CAD build for the part. Positions are in the model's coordinates, mm. A direction names the side the tool comes from. Give positions to 0.01 mm unless a question says otherwise; leave off trailing zeros. Write each loop counter-clockwise with the first axis right and the second up, starting at its lowest first coordinate (ties: lowest second). Pieces come first, ordered by that corner, then holes. Notation, with made-up numbers: (-21, 6.25) - (23, 6.25) arc R24 ccw to (23, 29.25) - close; hole circle Ø3 at (-10, -16). An arc over 180 degrees is marked (long way). Put each result on its own line as item: value. Start each with the question number.
1. Mould opens along Y. For faces 1 (the cylindrical face through (79.47, -0.8, 24.65)), 2 (the flat face through (-100.519, -2, 25)), 3 (the flat face through (-34, 48.316, 25)), 4 (the flat face through (-18, -42, 0)) say: +Y half, -Y half, draft (parallel to the pull), parting line (faces both ways), or undercut.
2. Cut at C-C on y = -16.5. List the corners of the cut face in (x, z).
3. Cut at B-B on z = 35. List the corners of the cut face in (x, y), and give its area (3 significant figures).
4. Wall check: line 1 (Y direction, x = -1.5, z = 34.5); line 2 (X direction, y = 0, z = 28); line 3 (X direction, y = 20.5, z = 42). Give the ranges that are in metal, low to high.
5. Drop flat-ended pins along their axis: pin 1 (5 mm diameter, centred on y = -15, z = 23, fed in from +X); pin 2 (25 mm diameter, centred on y = -8, z = 35.5, fed in from +X). Give the stop position or say it passes through.
6. Cut at A-A on x = -29. List the corners of the cut face in (y, z).
7. Tool access for faces 5 (the flat face through (-30, -41.684, 25)), 6 (the flat face through (-110.519, -1, 25)): list every direction of +Z, -Z, +X, -X, +Y, -Y with a clear straight run to the whole face (end or side of a thin tool).
from build123d import *

# Parameters (mm, degrees)
F1_DEPTH = 50


with BuildPart() as f1:
    # F0 (on Top) → F1 (new body)
    with BuildSketch(Plane.XY):
        Polygon((39.4807644188, 48.3160374686), (-110.5192355812, 48.3160374686), (-110.5192355812, -51.6839625314), (39.4807644188, -51.6839625314), (39.4807644188, -41.6839625314), (-100.5192355812, -41.6839625314), (-100.5192355812, 38.3160374686), (39.4807644188, 38.3160374686), align=None)
        with BuildLine():
            ThreePointArc((39.4807644188, -51.6839625314), (89.4807644188, -1.6839625314), (39.4807644188, 48.3160374686))
            Line((39.4807644188, 48.3160374686), (39.4807644188, 38.3160374686))
            ThreePointArc((39.4807644188, 38.3160374686), (79.4807644188, -1.6839625314), (39.4807644188, -41.6839625314))
            Line((39.4807644188, -41.6839625314), (39.4807644188, -51.6839625314))
        make_face()
    extrude(amount=F1_DEPTH)


solid = f1.part
Report:
1. face 1: undercut
1. face 2: undercut
1. face 3: +Y half
1. face 4: draft
2. outline: (-110.52, 0) - (-100.52, 0) - (-100.52, 50) - (-110.52, 50) - close; (76.64, 0) - (87.24, 0) - (87.24, 50) - (76.64, 50) - close
3. outline: (-110.52, -51.68) - (39.48, -51.68) arc R50 ccw to (39.48, 48.32) - (-110.52, 48.32) - close; hole (-100.52, -41.68) - (39.48, -41.68) arc R40 ccw to (39.48, 38.32) - (-100.52, 38.32) - close
3. area: 5,210 mm²
4. line 1: y = -51.68 to -41.68, 38.32 to 48.32
4. line 2: x = -110.52 to -100.52, 79.45 to 89.45
4. line 3: x = -110.52 to -100.52, 72.77 to 84.29
5. pin 1: stops at x = 88.3
5. pin 2: stops at x = 89.48
6. outline: (-51.68, 0) - (-41.68, 0) - (-41.68, 50) - (-51.68, 50) - close; (38.32, 0) - (48.32, 0) - (48.32, 50) - (38.32, 50) - close
7. face 5: +Z, -Z
7. face 6: +Z, -Z, -X, +Y, -Y
